Verification items for the finished model (mm, model axes). A direction names the side the tool comes from. Round coordinates to 2 decimals unless told otherwise and drop trailing zeros. Write each loop counter-clockwise with the first axis right and the second up, starting at its lowest first coordinate (ties: lowest second). Pieces come first, ordered by that corner, then holes. Notation, with made-up numbers: (7.5, 1) - (54.5, 1) arc R22 cw to (54.5, 28) - close; hole circle Ø5 at (44.25, 5.25). An arc over 180 degrees is marked (long way). Answer as a JSON object with one key per item and string values. Group by question number.
1) Thickness scan on line 1 (Y direction, x = 10.5, z = 3.1); line 2 (X direction, y = 9, z = 0); line 3 (Z direction, x = 5.75, y = 35). Record the ranges inside material, lowest first.
2) Mould release check, pull along X, two halves, no side actions. Record for faces 3 (the flat face through (2, 0, 1)), 4 (the flat face through (4.5, 28, 4)), 5 (the cylindrical face through (10.934, 27.548, 3.486)): +X half, -X half, draft (parallel to the pull), parting line (faces both ways), or undercut.
3) Section check C-C (y = 29.5). Enter the section's corners in (x, z).
4) Section check D-D (z = 0). Enter the section's corners in (x, y).
5) Set-up check for faces 1 (the cylindrical face through (15.359, 1.203, 3.486)), 2 (the cylindrical face through (-2.44, 27.62, 0.54)): record each of +Z, -Z, +X, -X, +Y, -Y from which the full face is reachable in a straight line by a thin tool's end or side.
6) Section check B-B (x = 10.5). Enter the section's corners in (y, z).
7) Go/stop test with flat-tipped pins: pin 1 Ø5 at (x, y) = (9, 23.5) entering from -Z; pin 2 Ø5 at (y, z) = (32.5, -1.5) entering from -X; pin 3 Ø0.6 at (y, z) = (29, 3.5) entering from -X. Record where each tip stops, or that it passes through.
8) Section check A-A (y = 7.5). Enter the section's corners in (x, z), then the cut area to 3 significant figures.
```python
from build123d import *

# Parameters (mm, degrees)
SKETCH_1_R          = 2.5
EXTRUDE_1_DEPTH     = 18.5
SKETCH_2_W          = 12
SKETCH_2_H          = 2
EXTRUDE_2_DEPTH     = 18.5
CUT_EXTRUDE_1_REACH = 43.113
SKETCH_3_R          = 2
FILLET_1_R          = 4
SKETCH_4_R          = 2.5
EXTRUDE_3_DEPTH     = 37


with BuildPart() as part:
    # 草图1 → 凸台-拉伸1 (new body)
    with BuildSketch(Plane(origin=(0, 0, 0), x_dir=(1, 0, 0), z_dir=(0, 1, 0))):
        with BuildLine():
            Line((0, -4.5), (16.5, -4.5))
            Line((16.5, -4.5), (16.5, -2.5))
            Line((16.5, -2.5), (3.741657387, -2.5))
            ThreePointArc((3.741657387, -2.5), (-2.121320344, 3.968626967), (0, -4.5))
        make_face()
        with Locations(Location((0, 0, 0), (0, 0, 270))):
            Circle(SKETCH_1_R, mode=Mode.SUBTRACT)
    extrude(amount=EXTRUDE_1_DEPTH)

    # 草图2 → 凸台-拉伸2 (add)
    with BuildSketch(Plane(origin=(0, 18.5, 0), x_dir=(1, 0, 0), z_dir=(0, 1, 0))):
        with Locations((10.5, -3.5)):
            Rectangle(SKETCH_2_W, SKETCH_2_H)
    extrude(amount=EXTRUDE_2_DEPTH)

    # 草图3 → 切除-拉伸1 (cut, up to next)
    with BuildSketch(Plane(origin=(0, 0, 2.5), x_dir=(-1, 0, 0), z_dir=(0, 0, -1)), mode=Mode.PRIVATE) as cut_extrude_1_sk1:
        with Locations((-10.5, 7.5)):
            Circle(SKETCH_3_R)
    cut_extrude_1_tool1 = extrude(cut_extrude_1_sk1.sketch, amount=-CUT_EXTRUDE_1_REACH, mode=Mode.PRIVATE) & part.part
    # 草图3 → 切除-拉伸1 (cut, up to next)
    with BuildSketch(Plane(origin=(0, 0, 2.5), x_dir=(-1, 0, 0), z_dir=(0, 0, -1)), mode=Mode.PRIVATE) as cut_extrude_1_sk2:
        with Locations((-10.5, 29.5)):
            Circle(SKETCH_3_R)
    cut_extrude_1_tool2 = extrude(cut_extrude_1_sk2.sketch, amount=-CUT_EXTRUDE_1_REACH, mode=Mode.PRIVATE) & part.part
    add(cut_extrude_1_tool1.solids().sort_by_distance((10.5, 7.5, 2.5))[0], mode=Mode.SUBTRACT)
    add(cut_extrude_1_tool2.solids().sort_by_distance((10.5, 29.5, 2.5))[0], mode=Mode.SUBTRACT)

    # 圆角1
    fillet_1_edges = [part.edges().sort_by_distance(p)[0] for p in [
        (16.5, 37, 3.5),
        (16.5, 0, 3.5),
    ]]
    fillet(fillet_1_edges, radius=FILLET_1_R)

    # 草图4 → 凸台-拉伸3 (add)
    with BuildSketch(Plane.XZ):
        with Locations(Location((0, 0, 0), (0, 0, 270))):
            Circle(SKETCH_4_R)
    extrude(amount=-EXTRUDE_3_DEPTH)


solid = part.part
```
Returned:
{
 "1": {"line 1": "0 to 5.5, 9.5 to 27.5, 31.5 to 37", "line 2": "-4.5 to 4.5", "line 3": "2.5 to 4.5"},
 "2": {"face 3": "draft", "face 4": "-X half", "face 5": "undercut"},
 "3": {"outline": "circle Ø5 at (0, 0); (4.5, 2.5) - (8.5, 2.5) - (8.5, 4.5) - (4.5, 4.5) - close; (12.5, 2.5) - (16.5, 2.5) - (16.5, 4.5) - (12.5, 4.5) - close"},
 "4": {"outline": "(-4.5, 0) - (4.5, 0) - (4.5, 18.5) - (2.5, 18.5) - (2.5, 37) - (-2.5, 37) - (-2.5, 18.5) - (-4.5, 18.5) - close"},
 "5": {"face 1": "+Z, -Z, +X, -Y", "face 2": "+Y"},
 "6": {"outline": "(0, 2.5) - (5.5, 2.5) - (5.5, 4.5) - (0, 4.5) - close; (9.5, 2.5) - (27.5, 2.5) - (27.5, 4.5) - (9.5, 4.5) - close; (31.5, 2.5) - (37, 2.5) - (37, 4.5) - (31.5, 4.5) - close"},
 "7": {"pin 1": "z = 2.5", "pin 2": "x = -2.5", "pin 3": "x = 4.5"},
 "8": {"outline": "(0, 4.5) arc R4.5 ccw (long way) to (3.74, 2.5) - (8.5, 2.5) - (8.5, 4.5) - close; (12.5, 2.5) - (16.5, 2.5) - (16.5, 4.5) - (12.5, 4.5) - close", "area": "83.4 mm2"}
}
